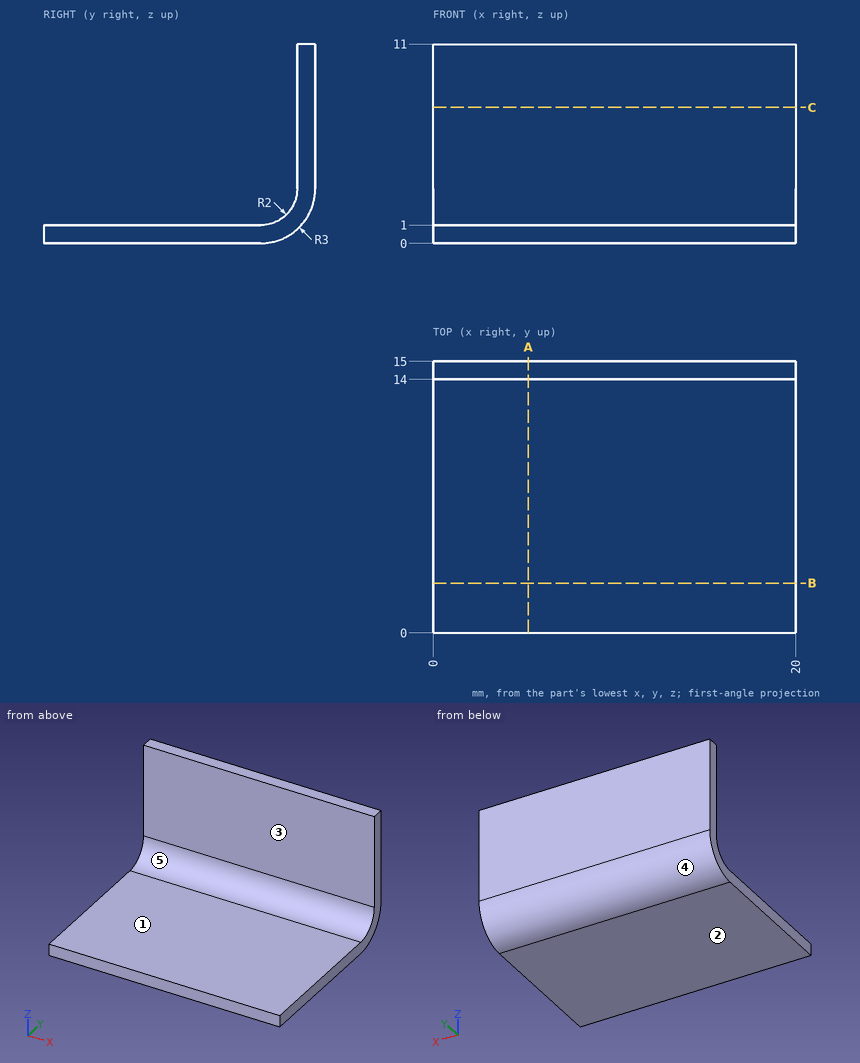
Verification items for this drawing (mm, ordinates from the low corner). A direction names the side the tool comes from. Coordinates: 2 decimals unless noted, no trailing zeros. Loops run counter-clockwise (first coordinate to the right, second up) from the corner with the lowest first, then second, coordinate; pieces in that order, holes last. Notation, with made-up numbers: (-20, -11) - (7, -11) arc R20 cw to (7, 19) - close; hole circle Ø6 at (51.5, 80.5). An arc over 180 degrees is marked (long way). One line per item, written item: value. Start each with the question number.
(1) Cross-section at B-B on y = 2.75. Enter the section's corners in (x, z).
(2) Depth check by flat-ended pin: P1, Ø8, axis at x = 4.5, y = 9.5, coming from the +Z side; P2, Ø6, axis at x = 7.5, y = 3.5, coming from the +Z side. Enter the tip coordinate at first touch or a pass-through.
(3) Material ranges on line 1 (Y direction, x = 17.25, z = 8.25); line 2 (Z direction, x = 15, y = 8.25); line 3 (Z direction, x = 1, y = 12.5), recorded low to high. Write a range as [from, to].
(4) Cross-section at C-C on z = 7.5. Enter the section's corners in (x, y), plus the area to 3 significant figures.
(5) Mould release check, pull along Z, two halves, no side actions. Record for the marked faces 3, 4 and 5: released by +Z, released by -Z, zero draft, split by the parting line, or undercut.
(6) Cross-section at A-A on x = 5.25. Enter the section's corners in (y, z), plus the area to 3 significant figures.
(7) Tool access check on the marked faces 1 and 2. Record the directions out of +Z, -Z, +X, -X, +Y, -Y that give a thin tool (end or side, any length) a straight path to the whole face; none if there is none.
Results below:
1. outline: (0, 0) - (20, 0) - (20, 1) - (0, 1) - close
2. P1: stops at z = 1.68
2. P2: stops at z = 1
3. line 1: y = [14, 15]
3. line 2: z = [0, 1]
3. line 3: z = [0.04, 1.06]
4. outline: (0, 14) - (20, 14) - (20, 15) - (0, 15) - close
4. area: 20.0 mm2
5. face 3: zero draft
5. face 4: released by -Z
5. face 5: released by +Z
6. outline: (0, 0) - (12, 0) arc R3 ccw to (15, 3) - (15, 11) - (14, 11) - (14, 3) arc R2 cw to (12, 1) - (0, 1) - close
6. area: 23.9 mm2
7. face 1: +Z, +X, -X, -Y
7. face 2: -Z, +X, -X, +Y, -Y
